from build123d import *

# Parameters (mm, degrees)
SKETCH1_R           = 4
SKETCH1_W           = 0.443674292
SKETCH1_H           = 0.606573965
SKETCH1_W_2         = 0.441272096
SKETCH1_W_3         = 0.539332563
SKETCH1_W_4         = 0.547504268
SKETCH1_W_5         = 0.686423262
SKETCH1_W_6         = 0.547504269
SKETCH1_W_7         = 0.607984695
SKETCH1_W_8         = 0.472854348
SKETCH1_W_9         = 0.501804613
SKETCH1_W_10        = 0.559705146
SKETCH1_W_11        = 0.321886919
SKETCH1_W_12        = 0.335329484
BOSS_EXTRUDE1_DEPTH = 36.8
SKETCH2_W           = 33.453118401
SKETCH2_H           = 26.8
CUT_EXTRUDE1_DEPTH  = 45
SCALE1_SCALE        = 0.7
BOSS_EXTRUDE2_DEPTH = 25.76


with BuildPart() as part:
    # Sketch1 → Boss-Extrude1 (new body)
    # profile 1 of 15: a face of its own
    with BuildSketch(Plane.XY):
        with BuildLine():
            ThreePointArc((-2.487228681, 2.47588145), (-1.643417841, 0.836304882), (0, 0))
            Line((0, 0), (42.98, -6.863043607))
            ThreePointArc((42.98, -6.863043607), (45.517837276, -6.94186018), (47.993719609, -6.378977628))
            ThreePointArc((47.993719609, -6.378977628), (70.945368499, -4.618817082), (91.44683801, -15.086199743))
            ThreePointArc((91.44683801, -15.086199743), (93.970071754, -16.788756754), (96.888617808, -17.653336321))
            Line((96.888617808, -17.653336321), (96.888617808, -17.138033163))
            Line((96.888617808, -17.138033163), (97.372163904, -17.138033163))
            Line((97.372163904, -17.138033163), (97.653484824, -17.138033163))
            Line((97.653484824, -17.138033163), (98.160101984, -17.138033163))
            Line((98.160101984, -17.138033163), (98.378364418, -17.138033163))
            Line((98.378364418, -17.138033163), (98.82203871, -17.138033163))
            Line((98.82203871, -17.138033163), (99.050846464, -17.138033163))
            Line((99.050846464, -17.138033163), (99.49211856, -17.138033163))
            Line((99.49211856, -17.138033163), (99.769956547, -17.138033163))
            Line((99.769956547, -17.138033163), (100.30928911, -17.138033163))
            Line((100.30928911, -17.138033163), (100.521753453, -17.138033163))
            Line((100.521753453, -17.138033163), (101.069257721, -17.138033163))
            Line((101.069257721, -17.138033163), (101.191833303, -17.138033163))
            Line((101.191833303, -17.138033163), (101.878256565, -17.138033163))
            Line((101.878256565, -17.138033163), (102.04986238, -17.138033163))
            Line((102.04986238, -17.138033163), (102.597366649, -17.138033163))
            Line((102.597366649, -17.138033163), (102.713161539, -17.138033163))
            Line((102.713161539, -17.138033163), (103.321146234, -17.138033163))
            Line((103.321146234, -17.138033163), (103.504651325, -17.138033163))
            Line((103.504651325, -17.138033163), (103.977505673, -17.138033163))
            Line((103.977505673, -17.138033163), (104.180157536, -17.138033163))
            Line((104.180157536, -17.138033163), (104.681962149, -17.138033163))
            Line((104.681962149, -17.138033163), (104.855663746, -17.138033163))
            Line((104.855663746, -17.138033163), (105.415368892, -17.138033163))
            Line((105.415368892, -17.138033163), (105.543243667, -17.138033163))
            Line((105.543243667, -17.138033163), (105.878573151, -17.138033163))
            Line((105.878573151, -17.138033163), (105.984724127, -17.138033163))
            Line((105.984724127, -17.138033163), (106.306611046, -17.138033163))
            Line((106.306611046, -17.138033163), (106.306611046, -17.744607128))
            ThreePointArc((106.306611046, -17.744607128), (108.688292645, -16.568776189), (109.203004303, -13.963002303))
            Line((109.203004303, -13.963002303), (108.439636924, -11.134191555))
            ThreePointArc((108.439636924, -11.134191555), (108.267803288, -10.660099415), (108.018988687, -10.221486316))
            Line((108.018988687, -10.221486316), (98.378364418, 3.865502848))
            ThreePointArc((98.378364418, 3.865502848), (93.609207326, 9.293547423), (87.68053985, 13.423853614))
            Line((87.68053985, 13.423853614), (25.781983162, 46.262452549))
            ThreePointArc((25.781983162, 46.262452549), (18.966543391, 48.873228311), (11.72235753, 49.761001134))
            Line((11.72235753, 49.761001134), (5.64235753, 49.761001134))
            ThreePointArc((5.64235753, 49.761001134), (5.616565931, 49.760890264), (5.590776238, 49.760557663))
            ThreePointArc((5.590776238, 49.760557663), (1.019670875, 48.889839007), (-2.994529703, 46.536256857))
            ThreePointArc((-2.994529703, 46.536256857), (-6.872179638, 41.155169878), (-7.760495561, 34.582258733))
            ThreePointArc((-7.760495561, 34.582258733), (-7.750828994, 34.504551611), (-7.739137581, 34.427123255))
            Line((-7.739137581, 34.427123255), (-2.487228681, 2.47588145))
        make_face()
        with Locations((8.267526818, 9.561727541)):
            Circle(SKETCH1_R, mode=Mode.SUBTRACT)
        with Locations((3.948380067, 39.69588145)):
            Circle(SKETCH1_R, mode=Mode.SUBTRACT)
    # profile 2 of 15: a face of its own
    with BuildSketch(Plane.XY):
        with BuildLine():
            Line((96.888617808, -17.138033163), (96.888617808, -17.653336321))
            ThreePointArc((96.888617808, -17.653336321), (97.130063387, -17.683196177), (97.372163904, -17.707173622))
            Line((97.372163904, -17.707173622), (97.372163904, -17.138033163))
            Line((97.372163904, -17.138033163), (96.888617808, -17.138033163))
        make_face()
    # profile 3 of 15: a face of its own
    with BuildSketch(Plane.XY):
        with BuildLine():
            Line((97.653484824, -17.138033163), (97.653484824, -17.727590841))
            ThreePointArc((97.653484824, -17.727590841), (97.906687423, -17.739163166), (98.160101984, -17.744314442))
            Line((98.160101984, -17.744314442), (98.160101984, -17.138033163))
            Line((98.160101984, -17.138033163), (97.653484824, -17.138033163))
        make_face()
    # profile 4 of 15: a face of its own
    with BuildSketch(Plane.XY):
        with Locations((98.600201564, -17.441320146)):
            Rectangle(SKETCH1_W, SKETCH1_H)
    # profile 5 of 15: a face of its own
    with BuildSketch(Plane.XY):
        with Locations((99.271482512, -17.441320146)):
            Rectangle(SKETCH1_W_2, SKETCH1_H)
    # profile 6 of 15: a face of its own
    with BuildSketch(Plane.XY):
        with Locations((100.039622829, -17.441320146)):
            Rectangle(SKETCH1_W_3, SKETCH1_H)
    # profile 7 of 15: a face of its own
    with BuildSketch(Plane.XY):
        with Locations((100.795505587, -17.441320146)):
            Rectangle(SKETCH1_W_4, SKETCH1_H)
    # profile 8 of 15: a face of its own
    with BuildSketch(Plane.XY):
        with Locations((101.535044934, -17.441320146)):
            Rectangle(SKETCH1_W_5, SKETCH1_H)
    # profile 9 of 15: a face of its own
    with BuildSketch(Plane.XY):
        with Locations((102.323614515, -17.441320146)):
            Rectangle(SKETCH1_W_6, SKETCH1_H)
    # profile 10 of 15: a face of its own
    with BuildSketch(Plane.XY):
        with Locations((103.017153887, -17.441320146)):
            Rectangle(SKETCH1_W_7, SKETCH1_H)
    # profile 11 of 15: a face of its own
    with BuildSketch(Plane.XY):
        with Locations((103.741078499, -17.441320146)):
            Rectangle(SKETCH1_W_8, SKETCH1_H)
    # profile 12 of 15: a face of its own
    with BuildSketch(Plane.XY):
        with Locations((104.431059843, -17.441320146)):
            Rectangle(SKETCH1_W_9, SKETCH1_H)
    # profile 13 of 15: a face of its own
    with BuildSketch(Plane.XY):
        with Locations((105.135516319, -17.441320146)):
            Rectangle(SKETCH1_W_10, SKETCH1_H)
    # profile 14 of 15: a face of its own
    with BuildSketch(Plane.XY):
        with Locations((106.145667586, -17.441320146)):
            Rectangle(SKETCH1_W_11, SKETCH1_H)
    # profile 15 of 15: a face of its own
    with BuildSketch(Plane.XY):
        with Locations((105.710908409, -17.441320146)):
            Rectangle(SKETCH1_W_12, SKETCH1_H)
    extrude(amount=BOSS_EXTRUDE1_DEPTH)

    # Sketch2 → Cut-Extrude1 (cut)
    with BuildSketch(Plane(origin=(0, -40, 0), x_dir=(1, 0, 0), z_dir=(0, 1, 0))):
        with Locations((69.72027881, -18.4)):
            Rectangle(SKETCH2_W, SKETCH2_H)
    extrude(amount=CUT_EXTRUDE1_DEPTH, mode=Mode.SUBTRACT)


with BuildPart() as part_1:
    # Scale1: scaled about (39.860062577, 16.282698439, 18.4)
    add(part.part.scale(SCALE1_SCALE).moved(Location((11.958018773, 4.884809532, 5.52))))

    # Sketch3 → Boss-Extrude2 (add)
    with BuildSketch(Plane.XY.offset(31.28)):
        Polygon((10.216958697, 6.617926547), (12.543544787, -7.536415458), (86.372646506, -7.536415458), (86.372646506, -6.950234368), (60.81181541, 6.617926547), align=None)
    extrude(amount=-BOSS_EXTRUDE2_DEPTH)


solid = part_1.part
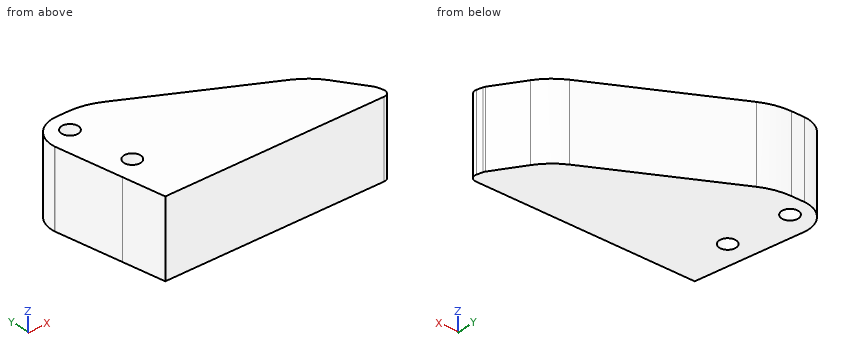
Verification items for the finished model (mm, model axes). Give positions to 0.01 mm unless a question says otherwise; leave off trailing zeros. Write each loop counter-clockwise with the first axis right and the second up, starting at its lowest first coordinate (ties: lowest second). Pieces come first, ordered by that corner, then holes.
(1) Cross-section at D-D (y = 12.5). Enter the section's corners in (x, z).
(2) Cross-section at C-C (z = 17.25). State how many separate pieces and enclosed holes the cut face has, plus the area to 3 significant figures.
(3) Material ranges on line 1 (X direction, y = 1.5, z = 25.25); line 2 (X direction, y = 30.5, z = 16.75); line 3 (Y direction, x = 71, z = 23.5), recorded low to high.
(4) Cross-section at B-B (x = 64.5). Enter the section's corners in (y, z), plus the area to 3 significant figures.
(5) Cross-section at A-A (y = 34). Enter the section's corners in (x, z).
(6) Gauge pin test, flat ends, axial feed: pin 1 (3.5 mm diameter, centred on x = 17.75, y = 11.58, fed in from -Z); pin 2 (8 mm diameter, centred on y = 6.5, z = 24, fed in from +X); pin 3 (4 mm diameter, centred on x = 73.5, z = 19, fed in from +Y); pin 4 (9.5 mm diameter, centred on x = 55.5, z = 18.5, fed in from +Y). Record the tip position at first contact, or that the pin passes through.
Worked out:
1. outline: (9.25, 5.52) - (15.1, 5.52) - (15.1, 31.28) - (9.25, 31.28) - close; (20.39, 5.52) - (76.13, 5.52) - (76.13, 31.28) - (20.39, 31.28) - close
2. separate pieces: 1
2. enclosed holes: 3
2. area: 2,500 mm2
3. line 1: x = 11.06 to 70.45, 72.47 to 84.99
3. line 2: x = 6.47 to 12.95, 16.49 to 42.76
3. line 3: y = -7.54 to 1.21, 8.38 to 15.52
4. outline: (-7.54, 5.52) - (18.97, 5.52) - (18.97, 31.28) - (-7.54, 31.28) - close; hole (4.66, 9.02) - (8.38, 9.02) - (8.38, 27.78) - (4.66, 27.78) - close
4. area: 613 mm2
5. outline: (7.28, 5.52) - (12.26, 5.52) - (12.26, 31.28) - (7.28, 31.28) - close; (17.19, 5.52) - (36.17, 5.52) - (36.17, 31.28) - (17.19, 31.28) - close
6. pin 1: passes through
6. pin 2: stops at x = 84.31
6. pin 3: stops at y = 15.25
6. pin 4: stops at y = 26.26
